The listing builds one solid part. Answer for the finished solid, in the listing's coordinates (mm). A direction names the side the tool comes from. Coordinates: 2 decimals unless noted, no trailing zeros. Write each loop counter-clockwise with the first axis right and the second up, starting at its lowest first coordinate (ties: lowest second). Pieces come first, ordered by that corner, then holes.
(1) Which of the six approach directions +Z, -Z, +X, -X, +Y, -Y give full straight-line access (tool end or side, diameter ignored) to faces 4 (the flat face through (-3.3, -0.5, 2.137)), 5 (the flat face through (3.961, -0.5, 0)), 6 (the flat face through (-0.617, -0.5, 2.8)), 7 (the flat face through (4.8, -0.5, -4.372)), 8 (the flat face through (0.2, -0.5, 3.703))?
(2) The part is cut by section A-A on y = 3.55. Determine the outline of the cut face in (x, z), plus the area to 3 significant figures.
(3) The part is cut by section C-C on z = -2. Determine the outline of the cut face in (x, y).
(4) Given P1, Ø0.8, axis at y = -0.5, z = -0.5, coming from the +X side; P2, Ø3, axis at x = -7.5, z = -1, coming from the -Y side; P3, Ø0.5, axis at y = -0.5, z = -0.5, coming from the -X side, each flat-ended and moving along its own axis, determine where each tip first touches the part or whether it passes through.
(5) The part is cut by section B-B on x = 12. Determine the outline of the cut face in (y, z), plus the area to 3 significant figures.
(6) Straight lines are drawn through the part: line 1 (Y direction, x = 4.5, z = 4.5); line 2 (Z direction, x = -13.5, y = 2.2); line 3 (Y direction, x = -14.5, z = 2.5). For each, find the intervals that lie inside material, in ascending order.
(7) The part is cut by section D-D on x = -14.5. Determine the outline of the cut face in (y, z).
(8) For a pull along X with two mould halves and no side action, classify faces 1 (the flat face through (0.2, -0.5, 1.852)), 2 (the flat face through (-2.705, -0.5, -0.2)), 3 (the flat face through (1.775, -0.5, -3.2)) as +X half, -X half, draft (parallel to the pull), parting line (faces both ways), or undercut.
from build123d import *

# Parameters (mm, degrees)
SKETCH1_W           = 35.56
SKETCH1_H           = 17.78
BOARD_DEPTH         = 1.57
SKETCH2_W           = 5
SKETCH2_H           = 8.06
MICROUSB_DEPTH      = 2.5
SKETCH3_W           = 2.2
SKETCH3_H           = 3.1
BUTTON_DEPTH        = 2.5
SKETCH4_W           = 1.388748629
SKETCH4_H           = 1.080137823
SKETCH4_W_2         = 1.028702689
SKETCH4_H_2         = 1.234443227
SKETCH4_W_3         = 1.131572957
SKETCH4_H_3         = 1.594489167
SKETCH4_W_4         = 0.720091882
SKETCH4_H_4         = 2.468886452
SKETCH4_W_5         = 1.74879457
SKETCH4_H_5         = 1.85166484
SKETCH4_W_6         = 0.925832419
SKETCH4_H_6         = 2.441025755
SKETCH4_W_7         = 0.76580757
SKETCH4_H_7         = 1.866499914
SKETCH4_W_8         = 1.080137823
SKETCH4_H_8         = 1.748794571
BOSS_EXTRUDE1_DEPTH = 1


with BuildPart() as part:
    # Sketch1 → Board (new body)
    with BuildSketch(Plane(origin=(0, 0, 0), x_dir=(1, 0, 0), z_dir=(0, 1, 0))):
        Rectangle(SKETCH1_W, SKETCH1_H)
    extrude(amount=BOARD_DEPTH)

    # Sketch2 → MicroUSB (add)
    with BuildSketch(Plane(origin=(0, 1.57, 0), x_dir=(1, 0, 0), z_dir=(0, 1, 0))):
        with Locations((-15.28, 0)):
            Rectangle(SKETCH2_W, SKETCH2_H)
    extrude(amount=MICROUSB_DEPTH)

    # Sketch3 → Button (add)
    with BuildSketch(Plane(origin=(0, 1.57, 0), x_dir=(1, 0, 0), z_dir=(0, 1, 0))):
        with Locations((12.19, 0)):
            Rectangle(SKETCH3_W, SKETCH3_H)
    extrude(amount=BUTTON_DEPTH)

    # Sketch4 → Boss-Extrude1 (add)
    with BuildSketch(Plane(origin=(0, 0, 0), x_dir=(1, 0, 0), z_dir=(0, 1, 0))):
        with Locations((-3.317566171, 4.371986427)):
            Rectangle(SKETCH4_W, SKETCH4_H)
        with Locations((1.260160794, 3.214695902)):
            Rectangle(SKETCH4_W_2, SKETCH4_H_2)
        with Locations((4.809185068, 3.574741842)):
            Rectangle(SKETCH4_W_3, SKETCH4_H_3)
        with Locations((3.60045941, 0)):
            Rectangle(SKETCH4_W_4, SKETCH4_H_4)
        with Locations((0.257175672, -2.777497259)):
            Rectangle(SKETCH4_W_5, SKETCH4_H_5)
        with Locations((-3.317566171, -3.357214086)):
            Rectangle(SKETCH4_W_6, SKETCH4_H_6)
        with Locations((-2.32174824, 0.229771707)):
            Rectangle(SKETCH4_W_7, SKETCH4_H_7)
        with Locations((3.240413468, -3.703329679)):
            Rectangle(SKETCH4_W_8, SKETCH4_H_8)
    extrude(amount=-BOSS_EXTRUDE1_DEPTH)


solid = part.part
Model answer:
1. face 4: -X, -Y
1. face 5: +Z, -Z, +X, -Y
1. face 6: +Z, -Z, -Y
1. face 7: -Z, +X, -Y
1. face 8: +Z, -Y
2. outline: (-17.78, -4.03) - (-12.78, -4.03) - (-12.78, 4.03) - (-17.78, 4.03) - close; (11.09, -1.55) - (13.29, -1.55) - (13.29, 1.55) - (11.09, 1.55) - close
2. area: 47.1 mm2
3. outline: (-17.78, 0) - (17.78, 0) - (17.78, 1.57) - (-12.78, 1.57) - (-12.78, 4.07) - (-17.78, 4.07) - close
4. P1: stops at x = 3.96
4. P2: stops at y = 0
4. P3: stops at x = -2.7
5. outline: (0, -8.89) - (1.57, -8.89) - (1.57, -1.55) - (4.07, -1.55) - (4.07, 1.55) - (1.57, 1.55) - (1.57, 8.89) - (0, 8.89) - close
5. area: 35.7 mm2
6. line 1: y = 0 to 1.57
6. line 2: z = -4.03 to 4.03
6. line 3: y = 0 to 4.07
7. outline: (0, -8.89) - (1.57, -8.89) - (1.57, -4.03) - (4.07, -4.03) - (4.07, 4.03) - (1.57, 4.03) - (1.57, 8.89) - (0, 8.89) - close
8. face 1: draft
8. face 2: -X half
8. face 3: undercut
